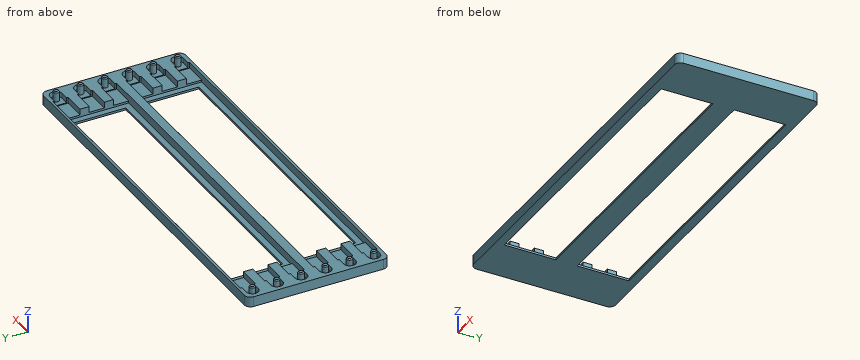
from build123d import *

# Parameters (mm, degrees)
F0_W      = 20
F0_H      = 70
F1_DEPTH  = 4
F3_DEPTH  = 2.6
F4_W      = 11
F4_H      = 7.5
F5_DEPTH  = 3
F6_R      = 1.45
F7_DEPTH  = 5
F8_SIZE   = 0.5
F10_W     = 75
F10_H     = 70
F9_W      = 20
F9_H      = 70
F11_DEPTH = 1
F14_W     = 150
F14_H     = 1.25
F14_H_2   = 4.5
F15_DEPTH = 4
F16_W     = 144
F16_H     = 25.5
F17_DEPTH = 1
F18_R     = 3


with BuildPart() as f1:
    # F0 (on Top) → F1 (new body)
    with BuildSketch(Plane.XY):
        with Locations((5, 30)):
            Rectangle(F0_W, F0_H)
    extrude(amount=F1_DEPTH)

    # F2 (on face) → F3 (cut)
    with BuildSketch(Plane.XY.offset(4)):
        with BuildLine():
            Line((15, 3), (0, 3))
            ThreePointArc((0, 3), (-3, 0), (0, -3))
            Line((0, -3), (15, -3))
            Line((15, -3), (15, 3))
        make_face()
        with BuildLine():
            Line((15, 15), (0, 15))
            ThreePointArc((0, 15), (-3, 12), (0, 9))
            Line((0, 9), (15, 9))
            Line((15, 9), (15, 15))
        make_face()
        with BuildLine():
            Line((15, 27), (0, 27))
            ThreePointArc((0, 27), (-3, 24), (0, 21))
            Line((0, 21), (15, 21))
            Line((15, 21), (15, 27))
        make_face()
        with BuildLine():
            Line((15, 39), (0, 39))
            ThreePointArc((0, 39), (-3, 36), (0, 33))
            Line((0, 33), (15, 33))
            Line((15, 33), (15, 39))
        make_face()
        with BuildLine():
            Line((15, 51), (0, 51))
            ThreePointArc((0, 51), (-3, 48), (0, 45))
            Line((0, 45), (15, 45))
            Line((15, 45), (15, 51))
        make_face()
        with BuildLine():
            Line((15, 63), (0, 63))
            ThreePointArc((0, 63), (-3, 60), (0, 57))
            Line((0, 57), (15, 57))
            Line((15, 57), (15, 63))
        make_face()
    extrude(amount=-F3_DEPTH, mode=Mode.SUBTRACT)

    # F4 (on face) → F5 (cut)
    with BuildSketch(Plane.XY.offset(4)):
        with Locations((9.5, 0)):
            Rectangle(F4_W, F4_H)
        Polygon((15, 15), (15, 15.75), (4, 15.75), (4, 15), (4, 8.25), (15, 8.25), (15, 9), align=None)
        Polygon((15, 27), (15, 27.75), (4, 27.75), (4, 27), (4, 20.25), (15, 20.25), (15, 21), align=None)
        Polygon((15, 39), (15, 39.75), (4, 39.75), (4, 39), (4, 32.25), (15, 32.25), (15, 33), align=None)
        Polygon((15, 51), (15, 51.75), (4, 51.75), (4, 51), (4, 44.25), (15, 44.25), (15, 45), align=None)
        Polygon((15, 63), (15, 63.75), (4, 63.75), (4, 63), (4, 56.25), (15, 56.25), (15, 57), align=None)
    extrude(amount=-F5_DEPTH, mode=Mode.SUBTRACT)

    # F6 (on face) → F7 (join)
    with BuildSketch(Plane.XY.offset(1.4)):
        Circle(F6_R)
        with Locations((0, 12)):
            Circle(F6_R)
        with Locations((0, 24)):
            Circle(F6_R)
        with Locations((0, 36)):
            Circle(F6_R)
        with Locations((0, 48)):
            Circle(F6_R)
        with Locations((0, 60)):
            Circle(F6_R)
    extrude(amount=F7_DEPTH)

    # F8
    f8_edges = [f1.edges().sort_by_distance(p)[0] for p in [
        (-1.45, 0, 6.4),
        (-1.45, 12, 6.4),
        (-1.45, 24, 6.4),
        (-1.45, 36, 6.4),
        (-1.45, 60, 6.4),
        (-1.45, 48, 6.4),
    ]]
    chamfer(f8_edges, length=F8_SIZE)

    # F10 (on face) + F9 (on face) → F11 (join)
    with BuildSketch(Plane(origin=(0, 0, 0), x_dir=(1, 0, 0), z_dir=(0, 0, -1))):
        with Locations((52.5, -30)):
            Rectangle(F10_W, F10_H)
    with BuildSketch(Plane(origin=(0, 0, 0), x_dir=(1, 0, 0), z_dir=(0, 0, -1))):
        with Locations((5, -30)):
            Rectangle(F9_W, F9_H)
    extrude(amount=F11_DEPTH)

    # F13: F1 across plane


with BuildPart() as f1_1:
    add(f1.part)
    add(f1.part.mirror(Plane(origin=(90, 30, -0.5), x_dir=(0, 1, 0), z_dir=(1, 0, 0))))

    # F14 (on face) → F15 (join, through all)
    with BuildSketch(Plane.XY.offset(4)):
        with Locations((90, -4.375)):
            Rectangle(F14_W, F14_H)
        with Locations((90, 30)):
            Rectangle(F14_W, F14_H_2)
        with Locations((90, 64.375)):
            Rectangle(F14_W, F14_H)
    extrude(amount=-F15_DEPTH)

    # F16 (on face) → F17 (cut, through all)
    with BuildSketch(Plane.XY):
        with Locations((90, 12)):
            Rectangle(F16_W, F16_H)
        with Locations((90, 48)):
            Rectangle(F16_W, F16_H)
    extrude(amount=-F17_DEPTH, mode=Mode.SUBTRACT)

    # F18
    f18_edges = [f1_1.edges().sort_by_distance(p)[0] for p in [
        (-5, -5, 1.5),
        (185, -5, 1.5),
        (185, 65, 1.5),
        (-5, 65, 1.5),
    ]]
    fillet(f18_edges, radius=F18_R)


solid = f1_1.part
Geometry check sheet. Reference: the model listing, model coordinates, mm. Coordinates: 2 decimals unless noted, no trailing zeros. Order: outer loops, then holes, each group sorted by start corner. A loop starts at its lowest first (then second) coordinate and runs counter-clockwise, first axis right, second up. Notation, with made-up numbers: M 67.5,76 L 77.5,76 A37 cw 77.5,115 Z; hole C 55.5,-15 d3. An arc over 180 degrees is marked long. Use CSV: the item, a comma, the result in double quotes.
Item 1: Cross-section at A-A on x = 31.5. Record the cut outline in (y, z).
Returned:
outline,"M -5,-1 L -0.75,-1 L -0.75,0 L -3.75,0 L -3.75,4 L -5,4 Z; M 24.75,-1 L 35.25,-1 L 35.25,0 L 32.25,0 L 32.25,4 L 27.75,4 L 27.75,0 L 24.75,0 Z; M 60.75,-1 L 65,-1 L 65,4 L 63.75,4 L 63.75,0 L 60.75,0 Z"
Item 2: Gauge pin test, flat end, axial feed: pin 1 Ø2 at (x, y) = (12, 24) entering from +Z. Record the tip position at first contact, or that the pin passes through.
Returned:
pin 1,"stops at z = 1"
Item 3: Thickness scan on line 1 along Y through (x, z) = (161.5, 2); line 2 along X through (y, z) = (54, 1.25); line 3 along Z through (x, y) = (27, 32). Record the ranges inside material, lowest first.
Returned:
line 1,"y = -5 to -3.75, 27.75 to 32.25, 63.75 to 65"
line 2,"x = -5 to 15, 165 to 185"
line 3,"z = -1 to 4"
